Part model, mm, in its own coordinate system. A direction names the side the tool comes from. Coordinates: 2 decimals unless noted, no trailing zeros. Loops run counter-clockwise (first coordinate to the right, second up) from the corner with the lowest first, then second, coordinate; pieces in that order, holes last. Notation, with made-up numbers: (62, 88) - (82, 88) arc R32 cw to (82, 114) - close; hole circle Ø2 at (-22, 39.25). An arc over 180 degrees is marked (long way). Answer as CSV lines item,"result".
from build123d import *

# Parameters (mm, degrees)
F0_W     = 14
F0_H     = 15.1035089948
F1_DEPTH = 17.78
F2_W     = 28
F2_H     = 15.1035089948
F3_DEPTH = 10
F3_TAPER = 4
F4_R     = 12.7
F5_W     = 1
F5_H     = 8.6030326784
F5_W_2   = 24
F5_H_2   = 4.5689390972
F5_R     = 1.5875
F6_DEPTH = 15.1045090948
F7_W     = 8.5285408422
F7_H     = 2.1393047646
F8_DEPTH = 7.62


# Not quite as in the source:
# - a feature names something its author has since deleted; it is built from what else it names


with BuildPart() as f1:
    # F0 (on Front) → F1 (new body)
    with BuildSketch(Plane.XZ):
        Polygon((-16, 0.5480427082), (-14, 0), (-14, 15.1035089948), (-16, 15.1035089948), align=None)
        with BuildLine():
            Line((-41.559, 7.5517544974), (-16, 0.5480427082))
            Line((-16, 0.5480427082), (-16, 15.1035089948))
            Line((-16, 15.1035089948), (-56.418, 15.1035089948))
            ThreePointArc((-56.418, 15.1035089948), (-65.3982561211, 11.3837651159), (-69.118, 2.4035089948))
            Line((-69.118, 2.4035089948), (-69.118, 0))
            Line((-69.118, 0), (-41.559, 7.5517544974))
        make_face()
        with Locations((-7, 7.5517544974)):
            Rectangle(F0_W, F0_H)
        with Locations((7, 7.5517544974)):
            Rectangle(F0_W, F0_H)
        with BuildLine():
            Line((16, 15.1035089948), (16, 0.5480427082))
            Line((16, 0.5480427082), (41.559, 7.5517544974))
            Line((41.559, 7.5517544974), (69.118, 0))
            Line((69.118, 0), (69.118, 2.4035089948))
            ThreePointArc((69.118, 2.4035089948), (65.3982561211, 11.3837651159), (56.418, 15.1035089948))
            Line((56.418, 15.1035089948), (16, 15.1035089948))
        make_face()
        Polygon((14, 15.1035089948), (14, 0), (16, 0.5480427082), (16, 15.1035089948), align=None)
    extrude(amount=F1_DEPTH)

    # F2 (on face) → F3 (join)
    with BuildSketch(Plane.XZ.offset(17.78)):
        with Locations((0, 7.5517544974)):
            Rectangle(F2_W, F2_H)
    extrude(amount=F3_DEPTH, taper=F3_TAPER)

    # F4
    f4_edges = [f1.edges().sort_by_distance(p)[0] for p in [
        (-41.559, -8.89, 7.551754),
    ]]
    fillet(f4_edges, radius=F4_R)

    # F5 (on face) → F6 (cut, through all)
    with BuildSketch(Plane(origin=(0, 0, 0), x_dir=(1, 0, 0), z_dir=(0, 0, -1))):
        with Locations((-12.5, 8.8704554364)):
            Rectangle(F5_W, F5_H)
        with Locations((0, 8.8704554364)):
            Rectangle(F5_W_2, F5_H)
        with Locations((0, 2.2844695486)):
            Rectangle(F5_W_2, F5_H_2)
        with Locations((12.5, 8.8704554364)):
            Rectangle(F5_W, F5_H)
        with Locations((0, 15.4564413242)):
            Rectangle(F5_W_2, F5_H_2)
        with Locations((0, 24.13)):
            Circle(F5_R)
    extrude(amount=-F6_DEPTH, mode=Mode.SUBTRACT)

    # F7 (on face) → F8 (cut)
    with BuildSketch(Plane.XZ.offset(27.78)):
        with Locations((0, 3.333498491)):
            Rectangle(F7_W, F7_H)
    extrude(amount=-F8_DEPTH, mode=Mode.SUBTRACT)


solid = f1.part
Q1. Saw through at B-B (x = 0). Count the separate pieces of the cut face and the enclosed holes in it, then the cut area to 3 significant figures.
Results:
separate pieces,"3"
enclosed holes,"0"
area,"90.0 mm^2"
Q2. Two-plate mould, pull along Z, no slides. Class faces 4 (the face through (0, -20.16, 3)), 5 (the face through (12, -2, 7)), 6 (the face through (65.5, -8.77, 11.28)): released by +Z, released by -Z, zero draft, split by the parting line, or undercut.
Results:
face 4,"undercut"
face 5,"zero draft"
face 6,"released by +Z"
Q3. Flat gauge pins, fed straight in: pin 1 (8.5 mm diameter, centred on x = 0, y = -23, fed in from -Z); pin 2 (6 mm diameter, centred on x = 18, y = -15, fed in from -Z); pin 3 (0.6 mm diameter, centred on x = 1, z = 3, fed in from -Y). Where does each tip first touch, or does it go through?
Results:
pin 1,"stops at z = 0.07"
pin 2,"stops at z = 0.27"
pin 3,"stops at y = -20.16"
Q4. Which spindle directions (+Z, -Z, +X, -X, +Y, -Y) get a long thin tool onto all of the face, cutting with end or side? Do faces 1 (the face through (12, -15, 7)), 2 (the face through (-57.19, -8.77, 3.27)), 3 (the face through (0, -26, 2.264)). Say none if no direction does.
Results:
face 1,"+Z, -Z, +Y"
face 2,"-Z, +Y, -Y"
face 3,"-Y"
Q5. Wall check: L1, parallel to Y at x = 0, z = 1.3; L2, parallel to Y at x = -5, z = 7.5; L3, parallel to X at y = -11.75, z = 10.75. Give the ranges that are in metal, low to high.
Results:
L1,"y = -27.78 to -25.72, -22.54 to -17.74"
L2,"y = -27.78 to -17.74"
L3,"x = -65.99 to -13, 13 to 65.99"
Q6. Saw through at A-A (y = -5.75). Give the cut face in (x, z).
Results:
outline,"(-69.12, 0) - (-44.92, 6.63) arc R12.7 cw to (-38.2, 6.63) - (-14, 0) - (-13, 0) - (-13, 15.1) - (-56.42, 15.1) arc R12.7 ccw to (-69.12, 2.4) - close; (13, 0) - (14, 0) - (41.56, 7.55) - (69.12, 0) - (69.12, 2.4) arc R12.7 ccw to (56.42, 15.1) - (13, 15.1) - close"
